```python
from build123d import *

# Parameters (mm, degrees)
SKETCH1_W                      = 393.7
SKETCH1_H                      = 127
BOSS_EXTRUDE1_DEPTH            = 6.35
F_10_CLEARANCE_HOLE1_D         = 4.9784
BOSS_EXTRUDE2_DEPTH            = 6.35
FILLET1_R                      = 6.35
F_8_CLEARANCE_HOLE1_D          = 4.3053
SKETCH11_W                     = 114.3
SKETCH11_H                     = 25.4
CUT_EXTRUDE1_DEPTH             = 226.28847424
F_5_16_0_3125_DIAMETER_HOLE1_D = 7.9375


with BuildPart() as part:
    # Sketch1 → Boss-Extrude1 (new body)
    with BuildSketch(Plane.XY):
        Rectangle(SKETCH1_W, SKETCH1_H)
    extrude(amount=BOSS_EXTRUDE1_DEPTH)

    # 10 Clearance Hole1 (through all)
    with Locations(Plane.XY.offset(6.35)):
        with Locations((-91.44, 27.94), (-91.44, -27.94), (91.44, 27.94), (91.44, -27.94), (-91.44, 0), (91.44, 0)):
            Hole(F_10_CLEARANCE_HOLE1_D / 2)

    # Sketch10 → Boss-Extrude2 (add)
    with BuildSketch(Plane.XY.offset(6.35)):
        Polygon((-152.4, 96.68304999), (-152.4, 63.5), (-139.7, 63.5), (-139.7, 96.68304999), (0, 96.68304999), (0, 109.38304999), (-146.05, 109.38304999), (-152.4, 109.38304999), align=None)
        Polygon((139.7, 96.68304999), (139.7, 63.5), (152.4, 63.5), (152.4, 109.38304999), (0, 109.38304999), (0, 96.68304999), align=None)
    extrude(amount=-BOSS_EXTRUDE2_DEPTH)

    # Fillet1
    fillet1_edges = [part.edges().sort_by_distance(p)[0] for p in [
        (139.7, 96.68304999, 3.175),
        (-139.7, 96.68304999, 3.175),
        (-139.7, 63.5, 3.175),
        (-152.4, 63.5, 3.175),
        (-152.4, 109.38304999, 3.175),
        (152.4, 109.38304999, 3.175),
        (152.4, 63.5, 3.175),
        (139.7, 63.5, 3.175),
    ]]
    fillet(fillet1_edges, radius=FILLET1_R)

    # 8 Clearance Hole1 (through all)
    with Locations(Plane.XY.offset(6.35)):
        with Locations((-147.828, 31.115), (-147.828, -31.115), (147.828, 18.415), (147.828, -18.415)):
            Hole(F_8_CLEARANCE_HOLE1_D / 2)

    # Sketch11 → Cut-Extrude1 (cut, through all)
    with BuildSketch(Plane.XY.offset(6.35)):
        with Locations((-63.5, -50.8)):
            Rectangle(SKETCH11_W, SKETCH11_H)
    extrude(amount=-CUT_EXTRUDE1_DEPTH, mode=Mode.SUBTRACT)

    # 5_16 _0.3125_ Diameter Hole1 (through all)
    with Locations(Plane.XY.offset(6.35)):
        with Locations((8.534908, -55.88)):
            Hole(F_5_16_0_3125_DIAMETER_HOLE1_D / 2)


solid = part.part
```
Geometry: final body of the model. Coordinates: model frame, mm. Coordinates: 2 decimals unless noted, no trailing zeros. Order: outer loops, then holes, each group sorted by start corner. A loop starts at its lowest first (then second) coordinate and runs counter-clockwise, first axis right, second up. Notation, with made-up numbers: (-7, 40) - (35, 40) arc R23 cw to (35, 77) - close; hole circle Ø7 at (-36.5, -25). An arc over 180 degrees is marked (long way). Return JSON: item names as keys, results as strings. Group by question number.
1. Pin query (flat end, axial travel): pin 1 (3 mm diameter, centred on x = -179, z = 4, fed in from +Y); pin 2 (7 mm diameter, centred on x = 8.53, y = -55.88, fed in from +Z). Return the tip coordinate at first contact, or that it passes through.
2. Cut plane B-B (x = -53). Output: boundary loops of the cut face in (y, z).
3. Material intervals for line 1 along Y through (x, z) = (8.5, 3.75); line 2 along Y through (x, z) = (91.44, 2); line 3 along Y through (x, z) = (-91.44, 4), sorted ascending. Write a range as [from, to].
4. Pull-direction query (X, two-part tool) for faces 1 (the face through (-3, 24, 0)), 2 (the face through (9.052, -51.945, 3.131)); classes: pulls with the +X half, pulls with the -X half, needs draft (parallel to the pull), parting line crosses it, or undercut.
5. Cut plane A-A (y = -47). Output: boundary loops of the cut face in (x, z), plus the area to 3 significant figures.
Resolved:
{
 "1": {"pin 1": "stops at y = 63.5", "pin 2": "passes through"},
 "2": {"outline": "(-38.1, 0) - (63.5, 0) - (63.5, 6.35) - (-38.1, 6.35) - close; (96.68, 0) - (109.38, 0) - (109.38, 6.35) - (96.68, 6.35) - close"},
 "3": {"line 1": "y = [-63.5, -59.85], [-51.91, 63.5], [96.68, 109.38]", "line 2": "y = [-63.5, -30.43], [-25.45, -2.49], [2.49, 25.45], [30.43, 63.5], [96.68, 109.38]", "line 3": "y = [-38.1, -30.43], [-25.45, -2.49], [2.49, 25.45], [30.43, 63.5], [96.68, 109.38]"},
 "4": {"face 1": "needs draft", "face 2": "undercut"},
 "5": {"outline": "(-196.85, 0) - (-120.65, 0) - (-120.65, 6.35) - (-196.85, 6.35) - close; (-6.35, 0) - (196.85, 0) - (196.85, 6.35) - (-6.35, 6.35) - close", "area": "1,770 mm²"}
}
